The model under review builds one solid part; all positions refer to its coordinate system, in mm. Round coordinates to 2 decimals unless told otherwise and drop trailing zeros. Order: outer loops, then holes, each group sorted by start corner. A loop starts at its lowest first (then second) coordinate and runs counter-clockwise, first axis right, second up. Notation, with made-up numbers: (52, 24) -> (108, 24) arc R16 ccw to (108, 34) -> close; hole circle Ø10 at (1.5, 1). An arc over 180 degrees is marked (long way). Put each result on its own line as item: value. Start each with the question number.
from build123d import *

# Parameters (mm, degrees)
F0_R     = 115
F0_R_2   = 2.5
F0_R_3   = 100
F1_DEPTH = 5


with BuildPart() as f1:
    # F0 (on Top) → F1 (new body)
    with BuildSketch(Plane.XY):
        Circle(F0_R)
        with Locations((-76.013979, -76.013979)):
            Circle(F0_R_2, mode=Mode.SUBTRACT)
        with BuildLine():
            ThreePointArc((0, -111.5), (-28.858324, -107.70073), (-55.75, -96.561833))
            ThreePointArc((-55.75, -96.561833), (-57.214102, -91.097731), (-51.75, -89.633629))
            ThreePointArc((-51.75, -89.633629), (-26.787771, -99.973323), (0, -103.5))
            ThreePointArc((0, -103.5), (4, -107.5), (0, -111.5))
        make_face(mode=Mode.SUBTRACT)
        with Locations((27.823047, -103.837026)):
            Circle(F0_R_2, mode=Mode.SUBTRACT)
        with Locations((103.837026, -27.823047)):
            Circle(F0_R_2, mode=Mode.SUBTRACT)
        with Locations((-103.837026, 27.823047)):
            Circle(F0_R_2, mode=Mode.SUBTRACT)
        with BuildLine():
            ThreePointArc((-96.561833, 55.75), (-78.842406, 78.842406), (-55.75, 96.561833))
            ThreePointArc((-55.75, 96.561833), (-50.285898, 95.097731), (-51.75, 89.633629))
            ThreePointArc((-51.75, 89.633629), (-73.185552, 73.185552), (-89.633629, 51.75))
            ThreePointArc((-89.633629, 51.75), (-95.097731, 50.285898), (-96.561833, 55.75))
        make_face(mode=Mode.SUBTRACT)
        with Locations((-27.823047, 103.837026)):
            Circle(F0_R_2, mode=Mode.SUBTRACT)
        Circle(F0_R_3, mode=Mode.SUBTRACT)
        with BuildLine():
            ThreePointArc((111.5, 0), (107.5, -4), (103.5, 0))
            ThreePointArc((103.5, 0), (99.973323, 26.787771), (89.633629, 51.75))
            ThreePointArc((89.633629, 51.75), (91.097731, 57.214102), (96.561833, 55.75))
            ThreePointArc((96.561833, 55.75), (107.70073, 28.858324), (111.5, 0))
        make_face(mode=Mode.SUBTRACT)
        with Locations((76.013979, 76.013979)):
            Circle(F0_R_2, mode=Mode.SUBTRACT)
    extrude(amount=F1_DEPTH)


solid = f1.part
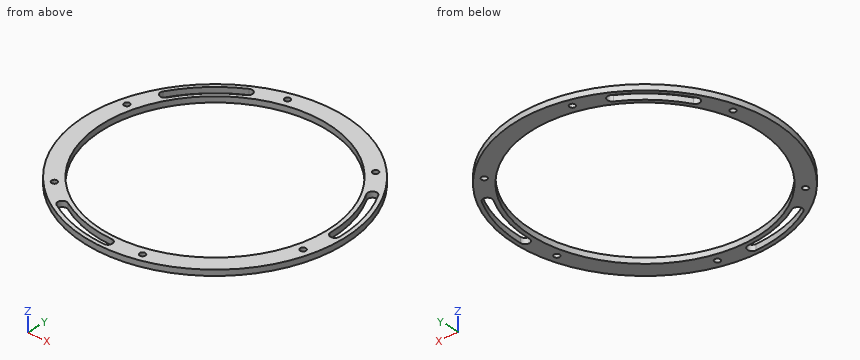
Q1. Wall thickness on probe 1 along Y at (x, z) = (-9, 4.25); probe 2 along Y at (x, z) = (-42, 4.25); probe 3 along X at (y, z) = (67, 2.65): over which ranges is each line inside the solid? List them lowest first. Write a range as [from, to].
Q2. Take a section at C-C on x = 53.5. Give the boundary of the cut face in (y, z).
Q3. Take a section at D-D on z = 0.75. State how many separate pieces and enclosed holes the cut face has, and give its area (3 significant figures).
Q4. Take a section at B-B on y = -49. Give the boundary of the cut face in (x, z), and give its area (3 significant figures).
Q5. Take a section at A-A on x = -15. Give the boundary of the cut face in (y, z).
Q6. Clearance check with flat-ended pins moving along their axes: pin 1 Ø1.5 at (y, z) = (-47, 1) entering from -X; pin 2 Ø1.5 at (y, z) = (61.5, 2.5) entering from -X; pin 3 Ø4 at (x, y) = (27.82, -103.84) entering from -Z; pin 4 Ø3 at (x, z) = (-56.5, 1) entering from -Y. State where each tip first meets the part, or that it passes through.
Calculated:
1. probe 1: y = [-114.65, -111.14], [-103.11, -99.59], [99.59, 114.65]
1. probe 2: y = [-107.06, -103.29], [-94.6, -90.75], [90.75, 107.06]
1. probe 3: x = [-93.47, -89.12], [-78.89, -74.24], [74.24, 93.47]
2. outline: (-101.8, 0) -> (-84.49, 0) -> (-84.49, 5) -> (-101.8, 5) -> close; (84.49, 0) -> (101.8, 0) -> (101.8, 5) -> (84.49, 5) -> close
3. separate pieces: 1
3. enclosed holes: 10
3. area: 8,510 mm²
4. outline: (-104.04, 0) -> (-87.17, 0) -> (-87.17, 5) -> (-104.04, 5) -> close; (87.17, 0) -> (104.04, 0) -> (104.04, 5) -> (87.17, 5) -> close
4. area: 169 mm²
5. outline: (-114.02, 0) -> (-110.49, 0) -> (-110.49, 5) -> (-114.02, 5) -> close; (-102.41, 0) -> (-98.87, 0) -> (-98.87, 5) -> (-102.41, 5) -> close; (98.87, 0) -> (114.02, 0) -> (114.02, 5) -> (98.87, 5) -> close
6. pin 1: stops at x = -105.29
6. pin 2: stops at x = -97.64
6. pin 3: passes through
6. pin 4: stops at y = -101
